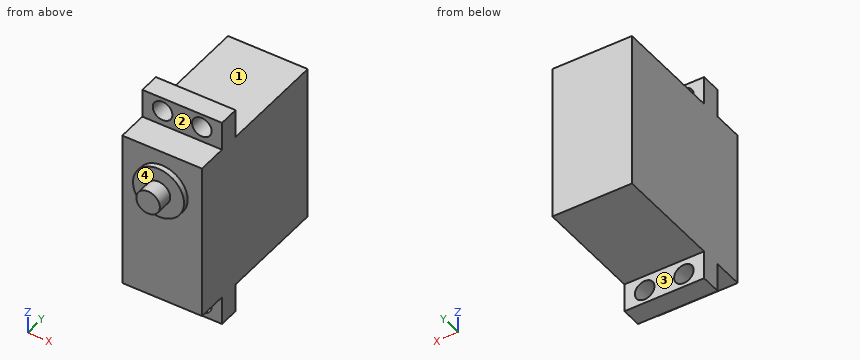
Autodesk Inventor part; units mm, degrees
ref_plane "YZ Plane" through (0, 0, 0) normal (1, 0, 0) x (0, 1, 0)
ref_plane "XZ Plane" through (0, 0, 0) normal (0, 1, 0) x (-1, 0, 0)
ref_plane "XY Plane" through (0, 0, 0) normal (0, 0, 1) x (1, 0, 0)
sketch "Skizze1" plane through (0, 0, 0) normal (0, 1, 0) x (-1, 0, 0)
  line L0 (10.15, 20.05) -> (-10.15, 20.05)
  line L1 (-10.15, 20.05) -> (-10.15, -20.05)
  line L2 (-10.15, -20.05) -> (10.15, -20.05)
  line L3 (10.15, -20.05) -> (10.15, 20.05)
  line L4 (14.21, 0) -> (-14.21, 0)
  line L5 (0, -28.07) -> (0, 28.07)
  point P0 (0, 0)
  dimension "d0" = 40.1
  dimension "d1" = 20.3
extrude "Extrusion1" add sketch "Skizze1" along normal blind 40.6
sketch "Skizze2" plane through (0, 0, 0) normal (0, -1, 0) x (1, 0, 0)
  circle A0 centre (0, 9.95) radius 6.5
  line L0 (10.15, -20.05) -> (-10.15, -20.05)
  line L1 (0, 28.07) -> (0, -28.07)
  point P0 (0, 0)
  dimension "d4" = 13
  dimension "d5" = 30
  dimension "d6" = 0
extrude "Extrusion2" add sketch "Skizze2" along normal blind 1.4
sketch "Skizze3" plane through (0, -1.4, 9.95) normal (0, -1, 0) x (1, 0, 0)
  circle A0 centre (0, 0) radius 3
  point P0 (0, -9.95)
  dimension "d9" = 6
extrude "Extrusion3" add sketch "Skizze3" along normal blind 4
sketch "Skizze4" plane through (-10.15, 0, 20.05) normal (0, 0, 1) x (1, 0, 0)
  line L0 (20.3, 7.7) -> (0, 7.7)
  line L1 (0, 7.7) -> (0, 12.9)
  line L2 (0, 12.9) -> (20.3, 12.9)
  line L3 (20.3, 12.9) -> (20.3, 7.7)
  line L4 (0, 0) -> (20.3, 0)
  line L5 (20.3, 0) -> (20.3, 40.6)
  point P0 (10.15, 0)
  point P1 (20.3, 10.3)
  dimension "d12" = 0
  dimension "d13" = 7.7
  dimension "d14" = 5.2
extrude "Extrusion4" add sketch "Skizze4" along normal blind 7.3
sketch "Skizze5" plane through (10.15, 0, -20.05) normal (0, 0, -1) x (-1, 0, 0)
  line L0 (20.3, 7.7) -> (0, 7.7)
  line L1 (0, 7.7) -> (0, 12.9)
  line L2 (0, 12.9) -> (20.3, 12.9)
  line L3 (20.3, 12.9) -> (20.3, 7.7)
  line L4 (0, 0) -> (20.3, 0)
  line L5 (20.3, 0) -> (20.3, 40.6)
  point P0 (10.15, 0)
  dimension "d17" = 0
  dimension "d20" = 7.7
  dimension "d21" = 5.2
extrude "Extrusion5" add sketch "Skizze5" along normal blind 7.3
sketch "Skizze6" plane through (-10.15, 7.7, 20.05) normal (0, -1, 0) x (1, 0, 0)
  circle A0 centre (15.15, 3.85) radius 2.5
  circle A1 centre (5.15, 3.85) radius 2.5
  circle A2 centre (15.15, -43.95) radius 2.5
  circle A3 centre (5.15, -43.95) radius 2.5
  line L0 (10.15, -58.34) -> (10.15, 18.24)
  line L1 (0, 7.3) -> (20.3, 7.3)
  line L2 (0, 0) -> (20.3, 0)
  line L3 (20.3, -40.1) -> (0, -40.1)
  point P0 (10.15, -20.05)
  dimension "d22" = 5
  dimension "d23" = 10
  dimension "d29" = 47.8
  dimension "d30" = 3.45
extrude "Extrusion6" cut sketch "Skizze6" against normal blind 7.3
properties part number "stepper_new"
Verification items for the finished model (mm, model axes). Face numbers are marked on the shaded views. A direction names the side the tool comes from. Round coordinates to 2 decimals unless told otherwise and drop trailing zeros. Loops run counter-clockwise (first coordinate to the right, second up) from the corner with the lowest first, then second, coordinate; pieces in that order, holes last. Notation, with made-up numbers: M 1,1.5 L 13,1.5 A26 cw 13,31.5 Z; hole C -15,47.25 d2. An arc over 180 degrees is marked long. Write each question's results on one line, items separated by ' | '.
1) Scan lines: L1, parallel to Z at x = 5, y = 9.4; L2, parallel to X at y = 11, z = -23; L3, parallel to Z at x = -6.5, y = 16. Record each from-to range of solid material in increasing order. Write a range as from..to.
Checks:
L1: z = -27.35..-26.4, -21.4..21.4, 26.4..27.35 | L2: x = -10.15..-7.33, -2.67..2.67, 7.33..10.15 | L3: z = -20.05..20.05
2) Section check B-B on y = 9. Record the boundary of the cut face in (x, z).
Checks:
outline: M -10.15,-27.35 L 10.15,-27.35 L 10.15,27.35 L -10.15,27.35 Z; hole C -5,-23.9 d5; hole C -5,23.9 d5; hole C 5,-23.9 d5; hole C 5,23.9 d5
3) Section check A-A on z = 23.9. Record the boundary of the cut face in (x, y), then the cut area to 3 significant figures.
Checks:
outline: M -10.15,7.7 L -7.5,7.7 L -7.5,12.9 L -10.15,12.9 Z; M -2.5,7.7 L 2.5,7.7 L 2.5,12.9 L -2.5,12.9 Z; M 7.5,7.7 L 10.15,7.7 L 10.15,12.9 L 7.5,12.9 Z | area: 53.6 mm2
4) Gauge pin test, flat ends, axial feed: P1, Ø6, axis at x = 5, z = -23.9, coming from the -Y side; P2, Ø3, axis at x = -4.5, z = 1, coming from the -Y side; P3, Ø5, axis at x = -1.5, y = 4, coming from the +Z side; P4, Ø8, axis at x = 1.5, z = -22, coming from the +Y side. Record the tip position at first contact, or that the pin passes through.
Checks:
P1: stops at y = 7.7 | P2: stops at y = 0 | P3: stops at z = 20.05 | P4: stops at y = 40.6
5) Section check C-C on x = -4.5. Record the boundary of the cut face in (y, z), then the cut area to 3 significant figures.
Checks:
outline: M -1.4,5.26 L 0,5.26 L 0,-20.05 L 7.7,-20.05 L 7.7,-21.45 L 12.9,-21.45 L 12.9,-20.05 L 40.6,-20.05 L 40.6,20.05 L 12.9,20.05 L 12.9,21.45 L 7.7,21.45 L 7.7,20.05 L 0,20.05 L 0,14.64 L -1.4,14.64 Z; M 7.7,-27.35 L 12.9,-27.35 L 12.9,-26.35 L 7.7,-26.35 Z; M 7.7,26.35 L 12.9,26.35 L 12.9,27.35 L 7.7,27.35 Z | area: 1,670 mm2
6) Section check D-D on z = 9.95. Record the boundary of the cut face in (x, y), then the cut area to 3 significant figures.
Checks:
outline: M -10.15,0 L -6.5,0 L -6.5,-1.4 L -3,-1.4 L -3,-5.4 L 3,-5.4 L 3,-1.4 L 6.5,-1.4 L 6.5,0 L 10.15,0 L 10.15,40.6 L -10.15,40.6 Z | area: 866 mm2
7) Access from +Z, -Z, +X, -X, +Y, -Y to the whole of each face (thin tool, end or side, straight path). Record for the marked faces 1, 2, 3 and 4.
Checks:
face 1: +Z, +X, -X, +Y | face 2: +Z, +X, -X, -Y | face 3: -Z, +X, -X, +Y | face 4: -Y
